Autodesk Inventor part; units mm, degrees
ref_plane "YZ Plane" through (0, 0, 0) normal (1, 0, 0) x (0, 1, 0)
ref_plane "XZ Plane" through (0, 0, 0) normal (0, 1, 0) x (-1, 0, 0)
ref_plane "XY Plane" through (0, 0, 0) normal (0, 0, 1) x (1, 0, 0)
sketch "Sketch1" plane through (0, 0, 0) normal (0, 1, 0) x (-1, 0, 0)
  line L0 (-1.27, 1.27) -> (1.27, 1.27)
  line L1 (1.27, 1.27) -> (1.27, -1.27)
  line L2 (1.27, -1.27) -> (-1.27, -1.27)
  line L3 (-1.27, -1.27) -> (-1.27, 1.27)
  line L4 (-1.27, 1.27) -> (1.27, -1.27) construction
  line L5 (1.27, 1.27) -> (-1.27, -1.27) construction
  point P0 (0, 0)
  dimension "d0" = 2.54
  dimension "d1" = 2.54
extrude "Extrusion1" add sketch "Sketch1" along normal blind 8.5
sketch "Sketch2" plane through (0, 8.5, 0) normal (0, 1, 0) x (1, 0, 0)
  line L0 (0.2, -0.2) -> (-0.2, -0.2)
  line L1 (-0.2, -0.2) -> (-0.2, 0.2)
  line L2 (-0.2, 0.2) -> (0.2, 0.2)
  line L3 (0.2, 0.2) -> (0.2, -0.2)
  line L4 (0.2, -0.2) -> (-0.2, 0.2) construction
  line L5 (-0.2, -0.2) -> (0.2, 0.2) construction
  point P0 (0, 0)
  dimension "d4" = 0.4
  dimension "d5" = 0.4
extrude "Extrusion2" cut sketch "Sketch2" against normal blind 5
chamfer "Chamfer1" distance 0.75 angle 45 4 edges at (0, 8.5, 0.2) (-0.2, 8.5, 0) (0, 8.5, -0.2) (0.2, 8.5, 0)
sketch "Sketch3" plane through (0, 0, 0) normal (0, -1, 0) x (1, 0, 0)
  line L0 (-0.2, 0.2) -> (0.2, 0.2)
  line L1 (0.2, 0.2) -> (0.2, -0.2)
  line L2 (0.2, -0.2) -> (-0.2, -0.2)
  line L3 (-0.2, -0.2) -> (-0.2, 0.2)
  line L4 (-0.2, 0.2) -> (0.2, -0.2) construction
  line L5 (0.2, 0.2) -> (-0.2, -0.2) construction
  point P0 (0, 0)
  dimension "d11" = 0.4
  dimension "d12" = 0.4
extrude "Extrusion3" add sketch "Sketch3" along normal blind 3
chamfer "Chamfer2" distance 0.074 distance2 0.5 1 edges at (-0.2, -3, 0) measured on face at (-0.0667, -3, 0.0667)
chamfer "Chamfer3" distance 0.074 distance2 0.5 1 edges at (0.2, -3, 0) measured on face at (-0.0173, -3, 0.0667)
chamfer "Chamfer4" distance 0.074 distance2 0.5 1 edges at (0, -3, 0.2) measured on face at (-0.042, -3, 0.0667)
chamfer "Chamfer5" distance 0.074 distance2 0.5 1 edges at (0, -3, -0.2) measured on face at (0.042, -3, -0.0913)
properties part number "FemaleHederPin"
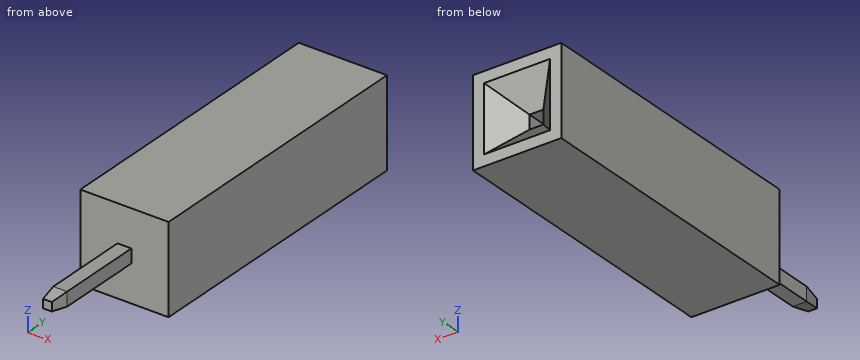
Verification items for the finished model (mm, model axes). Round coordinates to 2 decimals unless told otherwise and drop trailing zeros. Order: outer loops, then holes, each group sorted by start corner. A loop starts at its lowest first (then second) coordinate and runs counter-clockwise, first axis right, second up. Notation, with made-up numbers: (29, -11) -> (55, -11) arc R25 cw to (55, 9) -> close; hole circle Ø6 at (15.5, 23.5). An arc over 180 degrees is marked (long way). Put each result on its own line as item: value. Start each with the question number.
(1) Section check A-A (x = -0.4). Enter the section's corners in (y, z).
(2) Section check C-C (z = -0.55). Enter the section's corners in (x, y), then the cut area to 3 significant figures.
(3) Material ranges on line 1 along Y through (x, z) = (1.2, -0.7); line 2 along Y through (x, z) = (-0.3, -0.2), recorded low to high.
(4) Section check B-B (y = 4.5). Enter the section's corners in (x, z).
(5) Section check D-D (y = 8.25). Enter the section's corners in (x, z).
Completed:
1. outline: (0, -1.27) -> (8.5, -1.27) -> (8.5, -0.95) -> (7.95, -0.4) -> (7.95, 0.4) -> (8.5, 0.95) -> (8.5, 1.27) -> (0, 1.27) -> close
2. outline: (-1.27, 0) -> (1.27, 0) -> (1.27, 8.5) -> (0.95, 8.5) -> (0.55, 8.1) -> (-0.55, 8.1) -> (-0.95, 8.5) -> (-1.27, 8.5) -> close
2. area: 21.0 mm2
3. line 1: y = 0 to 8.5
3. line 2: y = 0 to 7.85
4. outline: (-1.27, -1.27) -> (1.27, -1.27) -> (1.27, 1.27) -> (-1.27, 1.27) -> close; hole (-0.2, -0.2) -> (0.2, -0.2) -> (0.2, 0.2) -> (-0.2, 0.2) -> close
5. outline: (-1.27, -1.27) -> (1.27, -1.27) -> (1.27, 1.27) -> (-1.27, 1.27) -> close; hole (-0.7, -0.7) -> (0.7, -0.7) -> (0.7, 0.7) -> (-0.7, 0.7) -> close
